CAD build for the part. Positions are in the model's coordinates, mm. A direction names the side the tool comes from. Coordinates: 2 decimals unless noted, no trailing zeros. Order: outer loops, then holes, each group sorted by start corner. A loop starts at its lowest first (then second) coordinate and runs counter-clockwise, first axis right, second up. Notation, with made-up numbers: M 58.5,52 L 63.5,52 A20 ccw 63.5,78 Z; hole C -21.75,79.25 d4. An arc over 180 degrees is marked long. Write item = value, one per line.
from build123d import *

# Parameters (mm, degrees)
BOSS_EXTRUDE1_DEPTH     = 107
CUT_EXTRUDE1_DEPTH      = 107
CUT_EXTRUDE1_DEPTH_BACK = 107
SKETCH2_W               = 29.989970731
SKETCH2_H               = 56.163122667


with BuildPart() as part:
    # Sketch1 → Boss-Extrude1 (new body)
    with BuildSketch(Plane.XY):
        Polygon((0, 0), (0, 3), (-36.192525263, 3), (-36.192525263, 29.472692743), (-26.142803298, 57.177331674), (-2.201948491, 122.954289658), (-5.021026354, 123.980350088), (-28.962436386, 58.201866633), (-39.192525263, 30), (-39.192525263, 0), align=None)
    extrude(amount=BOSS_EXTRUDE1_DEPTH)

    # Sketch2 → Cut-Extrude1 (cut, two sides: drawn at the far end of the back side and taken through both)
    with BuildSketch(Plane(origin=(0, 0, 0), x_dir=(0, 0, -1), z_dir=(1, 0, 0)).offset(-CUT_EXTRUDE1_DEPTH_BACK)):
        Polygon((-97.288221631, 0), (-97.288221631, 30.429310254), (-75.36242614, 30.429310254), (-75.36242614, 55.650312004), (-31.63757386, 55.650312004), (-31.63757386, 30.429310254), (-9.711778369, 30.429310254), (-9.711778369, 0), align=None)
        with Locations((-92.005014635, 95.898788755)):
            Rectangle(SKETCH2_W, SKETCH2_H)
        with Locations((-14.994985366, 95.898788755)):
            Rectangle(SKETCH2_W, SKETCH2_H)
    extrude(amount=CUT_EXTRUDE1_DEPTH + CUT_EXTRUDE1_DEPTH_BACK, mode=Mode.SUBTRACT)


solid = part.part
(1) Slice it at B-B, the plane x = -34. Write the cut outline in (y, z).
Evaluation:
outline = M 0,0 L 3,0 L 3,9.71 L 0,9.71 Z; M 0,97.29 L 3,97.29 L 3,107 L 0,107 Z; M 35.52,0 L 44.31,0 L 44.31,31.64 L 35.52,31.64 Z; M 35.52,75.36 L 44.31,75.36 L 44.31,107 L 35.52,107 Z
(2) Slice it at A-A, the plane y = 16. Write the cut outline in (x, z), then the cut area to 3 significant figures.
Evaluation:
outline = M -39.19,0 L -36.19,0 L -36.19,9.71 L -39.19,9.71 Z; M -39.19,97.29 L -36.19,97.29 L -36.19,107 L -39.19,107 Z
area = 58.3 mm²
(3) Wall check: line 1 (Y direction, x = -3, z = 9); line 2 (X direction, y = 89, z = 35.5); line 3 (X direction, y = 38.5, z = 7.5). Give the ranges that are in metal, low to high. Write a range as from..to.
Evaluation:
line_1 = 0..3
line_2 = -17.75..-14.56
line_3 = -36.11..-32.92
(4) Pull direction Z, two halves, no side cores. Call faces 6 (the face through (-39.193, 15, 5)), 7 (the face through (-37, 30.429, 21)), 8 (the face through (-27, 2, 9.712)), 9 (the face through (-37, 24, 0)): +Z half, -Z half, draft (parallel to the pull), parting line (faces both ways), or undercut.
Evaluation:
face_6 = draft
face_7 = undercut
face_8 = undercut
face_9 = -Z half
(5) Slice it at D-D, the plane z = 18. Write the cut outline in (x, y), then the cut area to 3 significant figures.
Evaluation:
outline = M -39.04,30.43 L -35.85,30.43 L -26.14,57.18 L -22.27,67.82 L -25.46,67.82 L -28.96,58.2 Z
area = 119 mm²
(6) Tool access for faces 1 (the face through (-39.193, 15, 102)), 2 (the face through (-36.193, 16, 5)), 3 (the face through (-24, 67.817, 92)), 4 (the face through (-24, 67.817, 15)), 5 (the face through (-28, 55.65, 54)): list every direction of +Z, -Z, +X, -X, +Y, -Y with a clear straight run to the whole face (end or side of a thin tool).
Evaluation:
face_1 = +Z, -Z, -X, +Y, -Y
face_2 = +Z, -Z, +X
face_3 = +Z, +X, -X, +Y
face_4 = -Z, +X, -X, +Y
face_5 = +X, -X, -Y
(7) Slice it at C-C, the plane x = -11. Write the cut outline in (y, z), then the cut area to 3 significant figures.
Evaluation:
outline = M 0,0 L 3,0 L 3,9.71 L 0,9.71 Z; M 0,97.29 L 3,97.29 L 3,107 L 0,107 Z; M 98.78,29.99 L 107.55,29.99 L 107.55,77.01 L 98.78,77.01 Z
area = 471 mm²
(8) Pin check, flat tips, straight feed: pin 1 Ø3 at (y, z) = (14, 3) entering from +X; pin 2 Ø5 at (y, z) = (35.5, 12.5) entering from +X; pin 3 Ø1 at (x, z) = (-38, 88) entering from -Y. Stop position of each tip, or through.
Evaluation:
pin_1 = -36.19
pin_2 = -33.1
pin_3 = 30.43
